Source: CAD feature listing. Evaluate the final solid. Frame: model axes, mm. A direction names the side the tool comes from. Give positions to 0.01 mm unless a question says otherwise; leave off trailing zeros. Write each loop counter-clockwise with the first axis right and the second up, starting at its lowest first coordinate (ties: lowest second). Pieces come first, ordered by that corner, then holes. Notation, with made-up numbers: (34, 67) -> (59, 67) arc R6 ccw to (59, 78) -> close; hole circle Ø6 at (9, 59). An arc over 180 degrees is marked (long way). Answer as a JSON object with one key per item and string values. Group by question number.
Item 1: Section query D-D on x = 4. Return the cut outline in (y, z).
Item 2: Access query for faces 1 (the face through (34, -2, -46.3)), 2 (the face through (28, -2.1, -8)), 3 (the face through (28, -1, -31)), 4 (the face through (58.7, -2, -44)), 5 (the face through (52.7, -1, -18)). Directions: +Z, -Z, +X, -X, +Y, -Y. A direction counts if a zero-diameter tool reaches every point of the face in a straight line with its end or side. Return the directions, or none.
Item 3: Pull-direction query (X, two-part tool) for faces 6 (the face through (34, -2, -41.3)), 7 (the face through (35, 6.9, -24)), 8 (the face through (25.7, -1, -24)); classes: pulls with the +X half, pulls with the -X half, needs draft (parallel to the pull), parting line crosses it, or undercut.
Item 4: Section query A-A on x = 27. Return the cut outline in (y, z).
Item 5: First-contact query: pin 1 Ø1 at (x, y) = (27, -1) entering from -Z; pin 2 Ø5 at (x, z) = (51, -23) entering from +Y; pin 3 Ø4.5 at (x, z) = (26.5, -25.5) entering from -Y; pin 4 Ø1.1 at (x, y) = (60, -0.5) entering from +Z. Flat tips, straight axial feed; report the tip coordinate or a pass-through.
Item 6: Section query B-B on z = -6. Return the cut outline in (x, y), plus the area to 3 significant figures.
Item 7: Section query C-C on z = -29. Return the cut outline in (x, y).
Item 8: Ray query, probe 1 along Z at (x, y) = (53.5, -2); probe 2 along Y at (x, z) = (10, -13); probe 3 along Y at (x, z) = (4, -20.5). Return the intervals inside material, ascending. Write a range as from..to.
from build123d import *

# Parameters (mm, degrees)
SKETCH1_W           = 65.7
SKETCH1_H           = 47.8
BOSS_EXTRUDE1_DEPTH = 7
SKETCH2_W           = 58
SKETCH2_H           = 43.2
CUT_EXTRUDE1_DEPTH  = 0.1
SKETCH3_W           = 13
SKETCH3_H           = 21
BOSS_EXTRUDE2_DEPTH = 1.4
SKETCH4_W           = 5.5
SKETCH4_H           = 8.5
BOSS_EXTRUDE3_DEPTH = 2.1
SKETCH5_W           = 4
SKETCH5_H           = 15
BOSS_EXTRUDE4_DEPTH = 1.3
SKETCH6_W           = 51
SKETCH6_H           = 5
BOSS_EXTRUDE5_DEPTH = 4


with BuildPart() as part:
    # Sketch1 → Boss-Extrude1 (new body)
    with BuildSketch(Plane(origin=(0, 0, 0), x_dir=(1, 0, 0), z_dir=(0, 1, 0))):
        with Locations((32.85, 23.9)):
            Rectangle(SKETCH1_W, SKETCH1_H)
    extrude(amount=BOSS_EXTRUDE1_DEPTH)

    # Sketch2 → Cut-Extrude1 (cut)
    with BuildSketch(Plane(origin=(0, 7, 0), x_dir=(1, 0, 0), z_dir=(0, 1, 0))):
        with Locations((34.95, 23.85)):
            Rectangle(SKETCH2_W, SKETCH2_H)
    extrude(amount=-CUT_EXTRUDE1_DEPTH, mode=Mode.SUBTRACT)

    # Sketch3 → Boss-Extrude2 (add)
    with BuildSketch(Plane.XZ):
        with Locations((59.2, -17.5)):
            Rectangle(SKETCH3_W, SKETCH3_H)
    extrude(amount=BOSS_EXTRUDE2_DEPTH)

    # Sketch4 → Boss-Extrude3 (add)
    with BuildSketch(Plane.XZ):
        with Locations((27.75, -7.75)):
            Rectangle(SKETCH4_W, SKETCH4_H)
    extrude(amount=BOSS_EXTRUDE3_DEPTH)

    # Sketch5 → Boss-Extrude4 (add)
    with BuildSketch(Plane.XZ):
        with Locations((27.7, -23.5)):
            Rectangle(SKETCH5_W, SKETCH5_H)
    extrude(amount=BOSS_EXTRUDE4_DEPTH)

    # Sketch6 → Boss-Extrude5 (add)
    with BuildSketch(Plane(origin=(0, 0, 0), x_dir=(-1, 0, 0), z_dir=(0, -1, 0))):
        with Locations((-33.2, 43.8)):
            Rectangle(SKETCH6_W, SKETCH6_H)
    extrude(amount=BOSS_EXTRUDE5_DEPTH)


solid = part.part
Worked answers:
{
 "1": {"outline": "(0, -47.8) -> (7, -47.8) -> (7, 0) -> (0, 0) -> close"},
 "2": {"face 1": "-Z, +X, -X, -Y", "face 2": "+Z, +X, -X, -Y", "face 3": "+X, -X, -Y", "face 4": "-Z, +X, -Y", "face 5": "+Z, -Y"},
 "3": {"face 6": "needs draft", "face 7": "undercut", "face 8": "pulls with the -X half"},
 "4": {"outline": "(-4, -46.3) -> (0, -46.3) -> (0, -47.8) -> (7, -47.8) -> (7, -45.45) -> (6.9, -45.45) -> (6.9, -2.25) -> (7, -2.25) -> (7, 0) -> (0, 0) -> (0, -3.5) -> (-2.1, -3.5) -> (-2.1, -12) -> (0, -12) -> (0, -16) -> (-1.3, -16) -> (-1.3, -31) -> (0, -31) -> (0, -41.3) -> (-4, -41.3) -> close"},
 "5": {"pin 1": "z = -46.3", "pin 2": "y = 6.9", "pin 3": "y = -1.3", "pin 4": "z = 0"},
 "6": {"outline": "(0, 0) -> (25, 0) -> (25, -2.1) -> (30.5, -2.1) -> (30.5, 0) -> (65.7, 0) -> (65.7, 7) -> (63.95, 7) -> (63.95, 6.9) -> (5.95, 6.9) -> (5.95, 7) -> (0, 7) -> close", "area": "466 mm^2"},
 "7": {"outline": "(0, 0) -> (25.7, 0) -> (25.7, -1.3) -> (29.7, -1.3) -> (29.7, 0) -> (65.7, 0) -> (65.7, 7) -> (63.95, 7) -> (63.95, 6.9) -> (5.95, 6.9) -> (5.95, 7) -> (0, 7) -> close"},
 "8": {"probe 1": "-46.3..-41.3", "probe 2": "0..6.9", "probe 3": "0..7"}
}
